Drawing for the job (mm, zero at the part's lowest x, y, z). Give positions to 0.01 mm unless a question says otherwise; leave off trailing zeros. Order: outer loops, then holes, each group sorted by start corner. A loop starts at its lowest first (then second) coordinate and runs counter-clockwise, first axis right, second up. Notation, with made-up numbers: (-39, -13) - (-24, -13) arc R28 cw to (-24, 5) - close; hole circle Ø1 at (82.25, 16). An arc over 180 degrees is marked (long way). Use a Markdown table: item, result. Add a question column.
(1) Flat gauge pins, fed straight in: pin 1 (2 mm diameter, centred on x = 703.5, z = 80, fed in from -Y); pin 2 (12 mm diameter, centred on x = 1239.5, z = 64.5, fed in from +Y); pin 3 (18 mm diameter, centred on x = 29.5, z = 162.5, fed in from +Y). Where does each tip first touch, or does it go through?
(2) Slice it at B-B (y = 336). Write the cut outline in (x, z), then the cut area to 3 significant figures.
(3) Slice it at C-C (x = 606). Write the cut outline in (y, z).
(4) Wall check: line 1 (X direction, y = 767.5, z = 220); line 2 (X direction, y = 118, z = 72); line 3 (X direction, y = 862, z = 33) (1 decimal). Give the ranges that are in metal, low to high.
(5) Slice it at A-A (z = 185). Write the cut outline in (x, y).
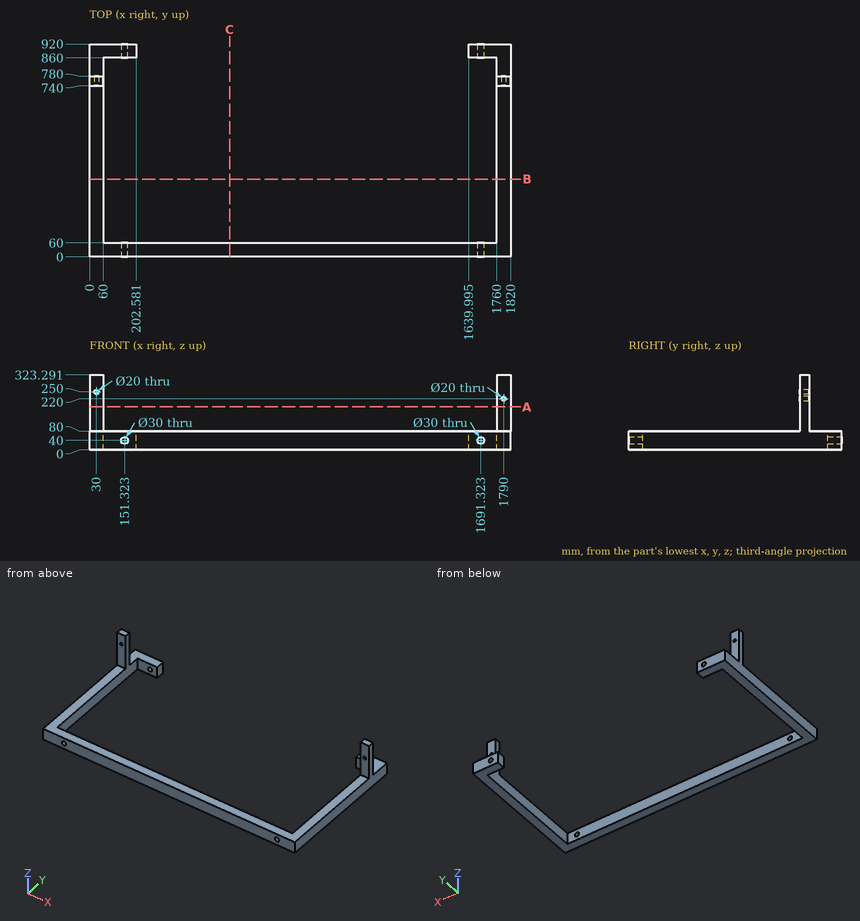
Solution:
| question | item | result |
|---|---|---|
| 1 | pin 1 | y = 0 |
| 1 | pin 2 | y = 60 |
| 1 | pin 3 | y = 780 |
| 2 | outline | (0, 0) - (60, 0) - (60, 80) - (0, 80) - close; (1760, 0) - (1820, 0) - (1820, 80) - (1760, 80) - close |
| 2 | area | 9,600 mm2 |
| 3 | outline | (0, 0) - (60, 0) - (60, 80) - (0, 80) - close |
| 4 | line 1 | 0 to 60, 1760 to 1780, 1800 to 1820 |
| 4 | line 2 | 0 to 60, 1760 to 1820 |
| 4 | line 3 | 0 to 138.1, 164.6 to 202.6, 1640 to 1678.1, 1704.6 to 1820 |
| 5 | outline | (0, 740) - (60, 740) - (60, 780) - (0, 780) - close; (1760, 740) - (1820, 740) - (1820, 780) - (1760, 780) - close |
